Can you work these out from the model? Positions are in its coordinate system, mm. A direction names the side the tool comes from. Give positions to 0.01 mm unless a question says otherwise; leave off trailing zeros. Write each loop counter-clockwise with the first axis right and the second up, starting at its lowest first coordinate (ties: lowest second). Pieces come first, ordered by that corner, then holes. Notation, with made-up numbers: (70.5, 3.25) -> (77.5, 3.25) arc R23 cw to (77.5, 22.25) -> close; hole circle Ø5 at (33, 25). An arc over 180 degrees is marked (long way). Answer as CSV lines item,"result". Start each with the question number.
1. If we section it at A-A on z = 36.75: Write out the boundary of the cut face in (x, y).
2. If we section it at D-D on x = 68.5: Write out the boundary of the cut face in (y, z).
3. If we section it at C-C on z = 24.5: Write out the boundary of the cut face in (x, y), plus the area to 3 significant figures.
4. On a 3-axis mill with a long thin cutter (end or side, diameter ignored), from which of +Z, -Z, +X, -X, +Y, -Y can I reach the whole of each face in a straight line? I mean faces 1 (the face through (107.245, -6.409, 3.521)), 2 (the face through (123, -7, 38)), 3 (the face through (122, -5, 35)), 4 (the face through (17, -7, 38)). Say none if no direction works.
5. I need wall thicknesses on line 1 (Z direction, x = 121, y = -9.5); line 2 (Z direction, x = 67, y = -2); line 3 (X direction, y = -9.5, z = 49). Which ranges of each line are inside material? Lowest first, please. Write a range as [from, to].
6. I'm going to push flat-ended pins straight in: P1, Ø3, axis at x = 104.5, y = -7.5, coming from the -Z side; P2, Ø6.5, axis at y = -9, z = 44.5, coming from the +X side; P3, Ø3, axis at y = -5, z = 56.75, coming from the +X side. Where does each tip first touch, or does it pass through?
7. If we section it at B-B on x = 5: Write out the boundary of the cut face in (y, z), plus the area to 3 significant figures.
8. If we mould it in two halves opening along Z, with no side actions, what happens to faces 5 (the face through (122.669, -6.591, 5.526)), 6 (the face through (102.87, -6.591, 67.773)), 7 (the face through (23.09, -6.59, 7.21))? For each: pulls with the +Z half, pulls with the -Z half, needs draft (parallel to the pull), parting line crosses it, or undercut.
```python
from build123d import *

# Parameters (mm, degrees)
F1_DEPTH = 13
F3_DEPTH = 25
F5_DEPTH = 25
F6_R     = 1.75
F7_DEPTH = 10
F8_R     = 1.75
F9_DEPTH = 25
F10_R    = 4
F11_R    = 2


with BuildPart() as f1:
    # F0 (on Front) → F1 (new body)
    with BuildSketch(Plane.XZ):
        Polygon((0, 75), (0, 0), (15, 0), (23, 7.5), (103, 7.5), (111, 0), (126, 0), (126, 75), (111, 75), (103, 67.5), (23, 67.5), (15, 75), align=None)
    extrude(amount=F1_DEPTH)

    # F2 (on face) → F3 (cut)
    with BuildSketch(Plane.XZ.offset(13)):
        with BuildLine():
            Line((116, 56), (21, 56))
            ThreePointArc((21, 56), (18.1715728753, 54.8284271247), (17, 52))
            Line((17, 52), (17, 23))
            ThreePointArc((17, 23), (18.1715728753, 20.1715728753), (21, 19))
            Line((21, 19), (116, 19))
            ThreePointArc((116, 19), (118.8284271247, 20.1715728753), (120, 23))
            Line((120, 23), (120, 52))
            ThreePointArc((120, 52), (118.8284271247, 54.8284271247), (116, 56))
        make_face()
    extrude(amount=-F3_DEPTH, mode=Mode.SUBTRACT)

    # F4 (on face) → F5 (cut)
    with BuildSketch(Plane.XZ.offset(13)):
        Polygon((126, 65), (123, 60), (123, 15), (126, 10), align=None)
    extrude(amount=-F5_DEPTH, mode=Mode.SUBTRACT)

    # F6 (on face) → F7 (cut)
    with BuildSketch(Plane.YZ.offset(123)):
        with Locations((-5, 36.75)):
            Circle(F6_R)
        with Locations((-5, 56.75)):
            Circle(F6_R)
    extrude(amount=-F7_DEPTH, mode=Mode.SUBTRACT)

    # F8 (on face) → F9 (cut)
    with BuildSketch(Plane.XZ.offset(13)):
        with Locations((5, 70)):
            Circle(F8_R)
        with Locations((5, 5)):
            Circle(F8_R)
        with Locations((121, 5)):
            Circle(F8_R)
        with Locations((121, 70)):
            Circle(F8_R)
    extrude(amount=-F9_DEPTH, mode=Mode.SUBTRACT)

    # F10
    f10_edges = [f1.edges().sort_by_distance(p)[0] for p in [
        (23, -6.5, 7.5),
        (103, -6.5, 7.5),
        (123, -6.5, 15),
        (123, -6.5, 60),
        (103, -6.5, 67.5),
        (23, -6.5, 67.5),
    ]]
    fillet(f10_edges, radius=F10_R)

    # F11
    f11_edges = [f1.edges().sort_by_distance(p)[0] for p in [
        (0, -6.5, 75),
        (0, -6.5, 0),
        (15, -6.5, 0),
        (111, -6.5, 0),
        (126, -6.5, 0),
        (126, -6.5, 10),
        (126, -6.5, 65),
        (126, -6.5, 75),
        (111, -6.5, 75),
        (15, -6.5, 75),
    ]]
    fillet(f11_edges, radius=F11_R)


solid = f1.part
```
Computed values:
1,outline,"(0, -13) -> (17, -13) -> (17, 0) -> (0, 0) -> close; (120, -13) -> (123, -13) -> (123, -6.75) -> (120, -6.75) -> close; (120, -3.25) -> (123, -3.25) -> (123, 0) -> (120, 0) -> close"
2,outline,"(-13, 7.5) -> (0, 7.5) -> (0, 19) -> (-13, 19) -> close; (-13, 56) -> (0, 56) -> (0, 67.5) -> (-13, 67.5) -> close"
3,outline,"(0, -13) -> (17, -13) -> (17, 0) -> (0, 0) -> close; (120, -13) -> (123, -13) -> (123, 0) -> (120, 0) -> close"
3,area,"260 mm2"
4,face 1,"-Z, +Y, -Y"
4,face 2,"+X, +Y, -Y"
4,face 3,"+X"
4,face 4,"+Y, -Y"
5,line 1,"z = [0, 3.25], [6.75, 68.25], [71.75, 75]"
5,line 2,"z = [7.5, 19], [56, 67.5]"
5,line 3,"x = [0, 17], [120, 123]"
6,P1,"stops at z = 4.69"
6,P2,"stops at x = 123"
6,P3,"stops at x = 113"
7,outline,"(-13, 0) -> (0, 0) -> (0, 3.25) -> (-13, 3.25) -> close; (-13, 6.75) -> (0, 6.75) -> (0, 68.25) -> (-13, 68.25) -> close; (-13, 71.75) -> (0, 71.75) -> (0, 75) -> (-13, 75) -> close"
7,area,"884 mm2"
8,face 5,"undercut"
8,face 6,"pulls with the +Z half"
8,face 7,"pulls with the -Z half"
